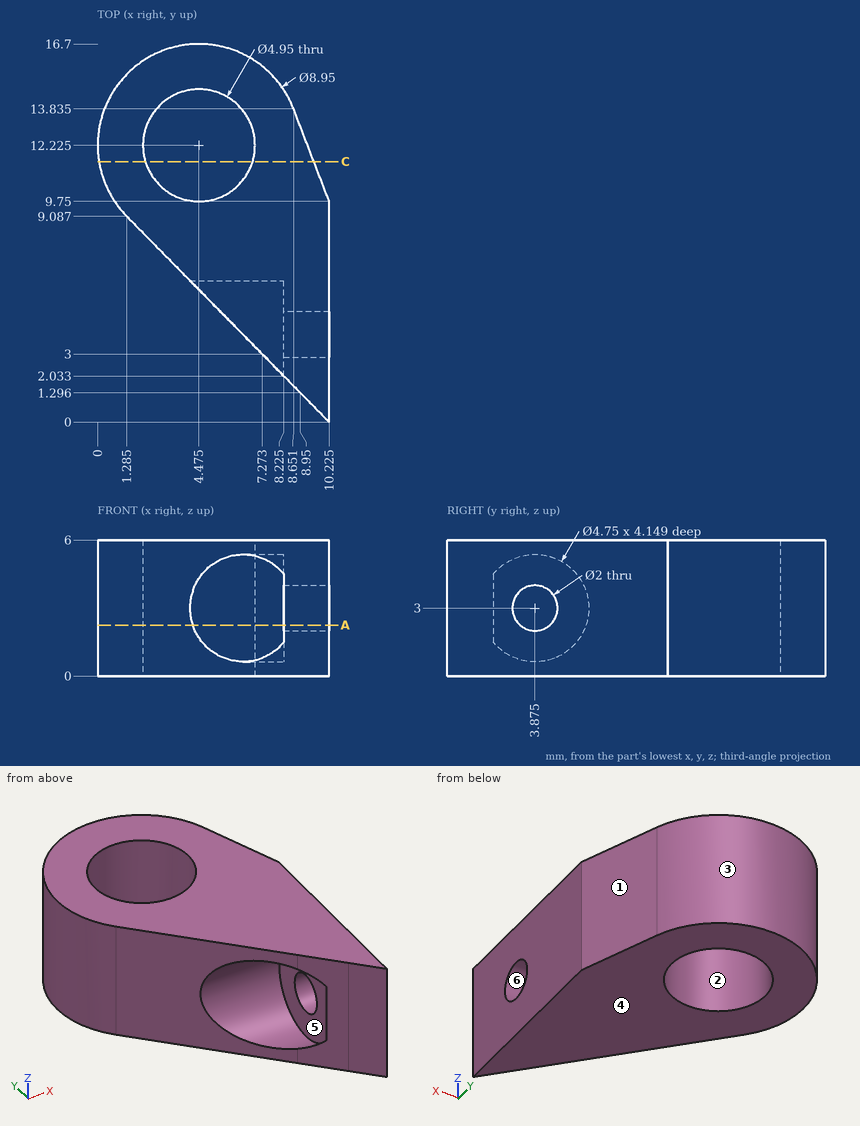
Study the drawing (mm; zero at the part's minimum x, y, z) and answer. A direction names the side the tool comes from. Round coordinates to 2 decimals unless told otherwise and drop trailing zeros. Order: outer loops, then holes, each group sorted by start corner. A loop starts at its lowest first (then second) coordinate and runs counter-clockwise, first axis right, second up. Notation, with made-up numbers: M -23.5,33 L 7.5,33 A31 ccw 7.5,66 Z; hole C 52.25,41 d4. An arc over 180 degrees is marked long. One line per item, written item: value.
Q1. Determine the mould class of the marked faces 1, 2, 3 and 4 for opening direction X: released by +X, released by -X, zero draft, split by the parting line, or undercut.
Derived:
face 1: released by +X
face 2: undercut
face 3: split by the parting line
face 4: zero draft
Q2. Flat-ended cylindrical pins translate along their axes: pin 1 (4.5 mm diameter, centred on x = 4.475, y = 12.225, fed in from -Z); pin 2 (1.3 mm diameter, centred on y = 4, z = 2.5, fed in from -X) (3 decimals); pin 3 (1.5 mm diameter, centred on y = 6.5, z = 1.5, fed in from -X). Find the tip coordinate at first contact, or state that the pin passes through.
Derived:
pin 1: through
pin 2: x = 8.225
pin 3: x = 3.09
Q3. Straight lines are drawn through the part: line 1 (Z direction, x = 7, y = 3.75); line 2 (Y direction, x = 4.75, z = 0.9) (1 decimal); line 3 (Y direction, x = 5.5, z = 4.55) (1 decimal). For each, find the intervals that lie inside material, in ascending order.
Derived:
line 1: 0 to 0.63, 5.37 to 6
line 2: 5.6 to 9.8, 14.7 to 16.7
line 3: 5.7 to 10, 14.5 to 16.6
Q4. Find section C-C on y = 11.5. Write down the section's boundary in (x, z).
Derived:
outline: M 0.06,0 L 2.11,0 L 2.11,6 L 0.06,6 Z; M 6.84,0 L 9.55,0 L 9.55,6 L 6.84,6 Z
Q5. For the marked faces 5 and 6, determine the directions among +Z, -Z, +X, -X, +Y, -Y from which every point of the face is accessible in a straight line to the end or side of a thin tool.
Derived:
face 5: -X
face 6: +X, -X
Q6. Find section A-A on z = 2.25. Give the number of separate pieces and of enclosed holes in the cut face.
Derived:
separate pieces: 2
enclosed holes: 1
